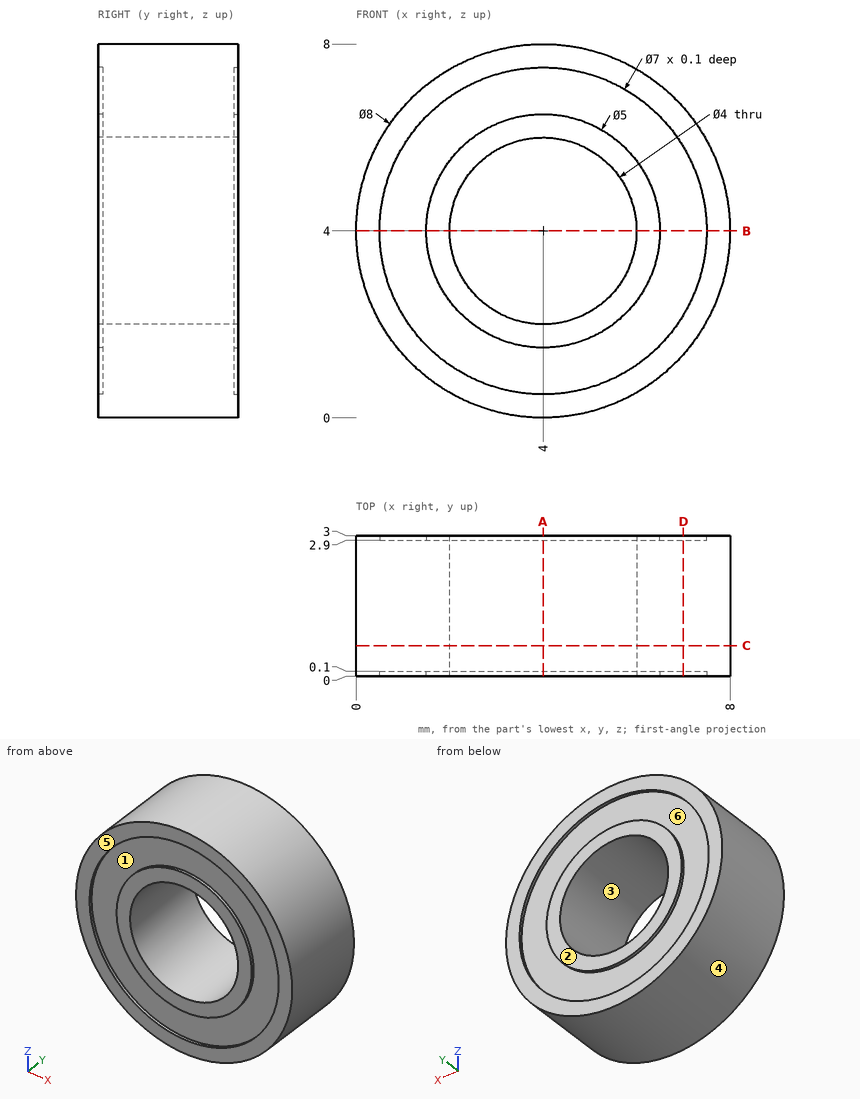
Part print with two shaded views. Sizes in mm from the minimum x, y, z corner. A direction names the side the tool comes from. Coordinates: 2 decimals unless noted, no trailing zeros. Write each loop counter-clockwise with the first axis right and the second up, starting at its lowest first coordinate (ties: lowest second). Pieces come first, ordered by that corner, then holes. Notation, with made-up numbers: (-19.75, 4) - (33.25, 4) arc R24 ccw to (33.25, 34) - close; hole circle Ø2 at (71.5, 34.25). An arc over 180 degrees is marked (long way). Use a Markdown table: item, result. Add a question column.
Item 1: Band-saw the part on A-A, the plane x = 4. Write the cut outline in (y, z).
Item 2: Band-saw the part on B-B, the plane z = 4. Write the cut outline in (x, y), and give its area (3 significant figures).
Item 3: Drop a flat-ended pin along its axis: pin 1 (3.5 mm diameter, centred on x = 3.5, z = 4.5, fed in from -Y). Give the stop position or say it passes through.
Item 4: Band-saw the part on C-C, the plane y = 0.65. Write the cut outline in (x, z), and give its area (3 significant figures).
Item 5: Drill centre lines: line 1 along Z through (x, y) = (4, 2.45); line 2 along Y through (x, z) = (1, 4.75); line 3 along Z through (x, y) = (4.5, 2.25). Where is each one in solid material? Low to high.
Item 6: Two-plate mould, pull along X, no slides. Class the marked faces 3, 4, 5 and 6: pulls with the +X half, pulls with the -X half, needs draft (parallel to the pull), parting line crosses it, or undercut.
Item 7: Band-saw the part on D-D, the plane x = 7. Write the cut outline in (y, z), and give its area (3 significant figures).
Item 8: 3-axis set-ups, long thin cutter, end or side, ignore diameter. For the marked faces 1 and 2: which of +Z, -Z, +X, -X, +Y, -Y reach the whole face in a straight line?
A:
| question | item | result |
|---|---|---|
| 1 | outline | (0, 0) - (3, 0) - (3, 0.5) - (2.9, 0.5) - (2.9, 1.5) - (3, 1.5) - (3, 2) - (0, 2) - (0, 1.5) - (0.1, 1.5) - (0.1, 0.5) - (0, 0.5) - close; (0, 6) - (3, 6) - (3, 6.5) - (2.9, 6.5) - (2.9, 7.5) - (3, 7.5) - (3, 8) - (0, 8) - (0, 7.5) - (0.1, 7.5) - (0.1, 6.5) - (0, 6.5) - close |
| 2 | outline | (0, 0) - (0.5, 0) - (0.5, 0.1) - (1.5, 0.1) - (1.5, 0) - (2, 0) - (2, 3) - (1.5, 3) - (1.5, 2.9) - (0.5, 2.9) - (0.5, 3) - (0, 3) - close; (6, 0) - (6.5, 0) - (6.5, 0.1) - (7.5, 0.1) - (7.5, 0) - (8, 0) - (8, 3) - (7.5, 3) - (7.5, 2.9) - (6.5, 2.9) - (6.5, 3) - (6, 3) - close |
| 2 | area | 11.6 mm² |
| 3 | pin 1 | stops at y = 0 |
| 4 | outline | circle Ø8 at (4, 4); hole circle Ø4 at (4, 4) |
| 4 | area | 37.7 mm² |
| 5 | line 1 | z = 0 to 2, 6 to 8 |
| 5 | line 2 | y = 0.1 to 2.9 |
| 5 | line 3 | z = 0.03 to 2.06, 5.94 to 7.97 |
| 6 | face 3 | undercut |
| 6 | face 4 | parting line crosses it |
| 6 | face 5 | needs draft |
| 6 | face 6 | undercut |
| 7 | outline | (0, 1.35) - (3, 1.35) - (3, 2.2) - (2.9, 2.2) - (2.9, 5.8) - (3, 5.8) - (3, 6.65) - (0, 6.65) - (0, 5.8) - (0.1, 5.8) - (0.1, 2.2) - (0, 2.2) - close |
| 7 | area | 15.2 mm² |
| 8 | face 1 | -Y |
| 8 | face 2 | +Z, -Z, +X, -X, +Y |
